from build123d import *

# Parameters (mm, degrees)
BOSS_EXTRUDE1_DEPTH = 1.7
BOSS_EXTRUDE3_DEPTH = 1.7
CUT_EXTRUDE1_DEPTH  = 1.7
SKETCH5_W           = 1
SKETCH5_H           = 1
BOSS_EXTRUDE4_DEPTH = 0.84


with BuildPart() as part:
    # Sketch1 → Boss-Extrude1 (new body)
    with BuildSketch(Plane(origin=(0, 0, 0), x_dir=(1, 0, 0), z_dir=(0, 1, 0))):
        with BuildLine():
            Line((-5, 8), (5, 8))
            ThreePointArc((5, 8), (6.414213562, 7.414213562), (7, 6))
            Line((7, 6), (7, -8))
            Line((7, -8), (-7, -8))
            Line((-7, -8), (-7, 6))
            ThreePointArc((-7, 6), (-6.414213562, 7.414213562), (-5, 8))
        make_face()
    extrude(amount=BOSS_EXTRUDE1_DEPTH)

    # Sketch3 → Boss-Extrude3 (add)
    with BuildSketch(Plane(origin=(0, 0, 0), x_dir=(1, 0, 0), z_dir=(0, 1, 0))):
        with BuildLine():
            Line((-6, 9), (6, 9))
            ThreePointArc((6, 9), (7.414213562, 8.414213562), (8, 7))
            Line((8, 7), (8, -9))
            Line((8, -9), (-8, -9))
            Line((-8, -9), (-8, 7))
            ThreePointArc((-8, 7), (-7.414213562, 8.414213562), (-6, 9))
        make_face()
    extrude(amount=BOSS_EXTRUDE3_DEPTH)

    # Sketch1<2> → Cut-Extrude1 (cut)
    with BuildSketch(Plane(origin=(0, 0, 0), x_dir=(1, 0, 0), z_dir=(0, 1, 0))):
        with BuildLine():
            Line((-5, 8), (5, 8))
            ThreePointArc((5, 8), (6.414213562, 7.414213562), (7, 6))
            Line((7, 6), (7, -8))
            Line((7, -8), (-7, -8))
            Line((-7, -8), (-7, 6))
            ThreePointArc((-7, 6), (-6.414213562, 7.414213562), (-5, 8))
        make_face()
    extrude(amount=CUT_EXTRUDE1_DEPTH, mode=Mode.SUBTRACT)

    # Sketch5 → Boss-Extrude4 (add)
    with BuildSketch(Plane(origin=(0, 1.7, 0), x_dir=(1, 0, 0), z_dir=(0, 1, 0))):
        with Locations((-4.5, 8.5)):
            Rectangle(SKETCH5_W, SKETCH5_H)
        with Locations((-7.5, -8.5)):
            Rectangle(SKETCH5_W, SKETCH5_H)
        with Locations((7.5, -8.5)):
            Rectangle(SKETCH5_W, SKETCH5_H)
        with Locations((4.5, 8.5)):
            Rectangle(SKETCH5_W, SKETCH5_H)
    extrude(amount=BOSS_EXTRUDE4_DEPTH)


solid = part.part
The listing builds one solid part. Answer for the finished solid, in the listing's coordinates (mm). A direction names the side the tool comes from. Round coordinates to 2 decimals unless told otherwise and drop trailing zeros. Order: outer loops, then holes, each group sorted by start corner. A loop starts at its lowest first (then second) coordinate and runs counter-clockwise, first axis right, second up. Notation, with made-up numbers: (28, 61) -> (60, 61) arc R24 cw to (60, 75) -> close; hole circle Ø1 at (-7.75, 47.25). An arc over 180 degrees is marked (long way). Put each result on its own line as item: value.
Q1. Which of the six approach directions +Z, -Z, +X, -X, +Y, -Y give full straight-line access (tool end or side, diameter ignored) to faces 1 (the flat face through (0, 1, -8)), 2 (the flat face through (-7.15, 1.7, -2.51)), 3 (the flat face through (-4, 2.1, -8.5))?
Results list:
face 1: +Y, -Y
face 2: -Z, -X, +Y
face 3: +Z, -Z, +Y
Q2. Section A-A, the plane y = 2.25 is taken. Write down the section's boundary in (x, z), and give its area (3 significant figures).
Results list:
outline: (-8, 8) -> (-7, 8) -> (-7, 9) -> (-8, 9) -> close; (-5, -9) -> (-4, -9) -> (-4, -8) -> (-5, -8) -> close; (4, -9) -> (5, -9) -> (5, -8) -> (4, -8) -> close; (7, 8) -> (8, 8) -> (8, 9) -> (7, 9) -> close
area: 4.00 mm^2
Q3. Determine the mould class of faces 4 (the flat face through (7.5, 2.1, 8)), 5 (the flat face through (0, 1, 8)), 6 (the flat face through (5, 2.1, -8.5)) for opening direction Z: pulls with the +Z half, pulls with the -Z half, needs draft (parallel to the pull), parting line crosses it, or undercut.
Results list:
face 4: pulls with the -Z half
face 5: undercut
face 6: needs draft
Q4. Section B-B, the plane z = -1.25 is taken. Write down the section's boundary in (x, y).
Results list:
outline: (-8, 0) -> (-7, 0) -> (-7, 1.7) -> (-8, 1.7) -> close; (7, 0) -> (8, 0) -> (8, 1.7) -> (7, 1.7) -> close
Q5. Section C-C, the plane x = 0 is taken. Write down the section's boundary in (y, z), and give its area (3 significant figures).
Results list:
outline: (0, -9) -> (1.7, -9) -> (1.7, -8) -> (0, -8) -> close; (0, 8) -> (1.7, 8) -> (1.7, 9) -> (0, 9) -> close
area: 3.40 mm^2
Q6. Consider line 1 along X through (y, z) = (1.4, -5.5); line 2 along Z through (x, y) = (-0.5, 0.7); line 3 along Z through (x, y) = (-4.25, 2.2). Determine where each line is inside the solid, lowest interval first.
Results list:
line 1: -8 to -7, 7 to 8
line 2: -9 to -8, 8 to 9
line 3: -9 to -8
Q7. Section D-D, the plane y = 0.4 is taken. Write down the section's boundary in (x, z), and give its area (3 significant figures).
Results list:
outline: (-8, -7) arc R2 ccw to (-6, -9) -> (6, -9) arc R2 ccw to (8, -7) -> (8, 9) -> (-8, 9) -> close; hole (-7, -6) arc R2 ccw to (-5, -8) -> (5, -8) arc R2 ccw to (7, -6) -> (7, 8) -> (-7, 8) -> close
area: 64.0 mm^2
Q8. Each of these flat-tipped pins is pushed along its axis until it touches: P1, Ø3.5, axis at x = 6.5, z = 0, coming from the +Y side; P2, Ø0.7, axis at y = 2.5, z = -8.5, coming from the +X side; P3, Ø0.9, axis at y = 2, z = -8.5, coming from the -X side. Where does it stop, or does it pass through?
Results list:
P1: y = 1.7
P2: x = 5
P3: x = -7.63
